Autodesk Inventor part; units mm, degrees
ref_plane "YZ Plane" through (0, 0, 0) normal (1, 0, 0) x (0, 1, 0)
ref_plane "XZ Plane" through (0, 0, 0) normal (0, 1, 0) x (-1, 0, 0)
ref_plane "XY Plane" through (0, 0, 0) normal (0, 0, 1) x (1, 0, 0)
sketch "Sketch1" plane through (0, 0, 0) normal (0, 0, 1) x (1, 0, 0)
  circle A0 centre (0, 0) radius 45.212
  dimension "d0" = 90.424
extrude "Extrusion1" add sketch "Sketch1" along normal blind 4.7625
sketch "Sketch6" plane through (0, 0, 4.7625) normal (0, 0, 1) x (1, 0, 0)
  circle A0 centre (12.446, -29.7561) radius 3.048
  point P0 (0, 0)
  dimension "d27" = 6.096
  dimension "d28" = 29.7561
  dimension "d29" = 12.446
extrude "Extrusion6" cut sketch "Sketch6" against normal blind 25.4
sketch "Sketch7" plane through (0, 0, 4.7625) normal (0, 0, 1) x (1, 0, 0)
  line L0 (0, 0) -> (21.4313, 37.12)
  line L1 (0, 0) -> (42.8625, 0) construction
  circle A0 centre (21.4313, 37.12) radius 1.7145
  circle A1 centre (-21.4312, 37.12) radius 1.7145
  circle A2 centre (-42.8625, 0) radius 1.7145
  circle A3 centre (-21.4313, -37.12) radius 1.7145
  circle A4 centre (21.4312, -37.12) radius 1.7145
  circle A5 centre (42.8625, 0) radius 1.7145
  dimension "d32" = 42.8625
  dimension "d33" = 60
  dimension "d34" = 3.429
  dimension "d37" = 360
extrude "Extrusion7" cut sketch "Sketch7" against normal blind 25.4
sketch "Sketch8" plane through (0, 0, 4.7625) normal (0, 0, 1) x (1, 0, 0)
  line L0 (0, 0) -> (0, 41.91)
  circle A0 centre (0, 41.91) radius 1.8415
  circle A1 centre (-36.2951, 20.955) radius 1.8415
  circle A2 centre (-36.2951, -20.955) radius 1.8415
  circle A3 centre (0, -41.91) radius 1.8415
  circle A4 centre (36.2951, -20.955) radius 1.8415
  circle A5 centre (36.2951, 20.955) radius 1.8415
  dimension "d41" = 41.91
  dimension "d42" = 3.683
  dimension "d45" = 360
extrude "Extrusion8" cut sketch "Sketch8" against normal blind 25.4
sketch "Sketch10" plane through (0, 0, 4.7625) normal (0, 0, 1) x (1, 0, 0)
  line L0 (0, 0) -> (39.3779, 10.5513)
  line L1 (0, 0) -> (40.767, 0) construction
  circle A0 centre (39.3779, 10.5513) radius 3.81
  line L2 (0, 0) -> (0, 16.2318)
  circle A1 centre (39.3779, -10.5513) radius 3.81
  circle A2 centre (-39.3779, 10.5513) radius 3.81
  circle A3 centre (-39.3779, -10.5513) radius 3.81
  line L3 (0, 0) -> (28.8266, 28.8266)
  line L4 (0, 0) -> (40.767, 0) construction
  circle A4 centre (28.8266, 28.8266) radius 3.81
  circle A5 centre (-28.8266, 28.8266) radius 3.81
  dimension "d49" = 40.767
  dimension "d50" = 15
  dimension "d51" = 7.62
  dimension "d68" = 40.767
  dimension "d69" = 45
  dimension "d70" = 7.62
extrude "Extrusion9" cut sketch "Sketch10" against normal blind 25.4 contours A0 | A1 | A2 | A3
sketch "Sketch11" plane through (0, 0, 4.7625) normal (0, 0, 1) x (1, 0, 0)
  circle A0 centre (-39.3779, 10.5513) radius 3.81
  circle A1 centre (39.3779, 10.5513) radius 3.81
  circle A2 centre (39.3779, -10.5513) radius 3.81
  circle A3 centre (-39.3779, -10.5513) radius 3.81
  circle A4 centre (36.2951, -20.955) radius 1.8415
  circle A5 centre (-36.2951, -20.955) radius 1.8415
  circle A6 centre (0, 41.91) radius 1.8415
  circle A7 centre (-36.2951, 20.955) radius 1.8415
  circle A8 centre (0, -41.91) radius 1.8415
  circle A9 centre (36.2951, 20.955) radius 1.8415
  circle A10 centre (21.4312, -37.12) radius 1.7145
  circle A11 centre (-42.8625, 0) radius 1.7145
  circle A12 centre (21.4313, 37.12) radius 1.7145
  circle A13 centre (-21.4312, 37.12) radius 1.7145
  circle A14 centre (-21.4313, -37.12) radius 1.7145
  circle A15 centre (42.8625, 0) radius 1.7145
  circle A16 centre (12.446, -29.7561) radius 3.048
  circle A17 centre (0, 0) radius 45.212
  circle A18 centre (0, 0) radius 25.4
  dimension "d54" = 50.8
extrude "Extrusion10" cut sketch "Sketch11" against normal blind 25.4 contours A18
sketch "Sketch12" plane through (0, 0, 4.7625) normal (0, 0, 1) x (1, 0, 0)
  circle A0 centre (0, 0) radius 25.4
  circle A1 centre (-39.3779, 10.5513) radius 3.81
  circle A2 centre (39.3779, 10.5513) radius 3.81
  circle A3 centre (39.3779, -10.5513) radius 3.81
  circle A4 centre (-39.3779, -10.5513) radius 3.81
  circle A5 centre (36.2951, -20.955) radius 1.8415
  circle A6 centre (-36.2951, -20.955) radius 1.8415
  circle A7 centre (0, 41.91) radius 1.8415
  circle A8 centre (-36.2951, 20.955) radius 1.8415
  circle A9 centre (0, -41.91) radius 1.8415
  circle A10 centre (36.2951, 20.955) radius 1.8415
  circle A11 centre (21.4312, -37.12) radius 1.7145
  circle A12 centre (-42.8625, 0) radius 1.7145
  circle A13 centre (21.4313, 37.12) radius 1.7145
  circle A14 centre (-21.4312, 37.12) radius 1.7145
  circle A15 centre (-21.4313, -37.12) radius 1.7145
  circle A16 centre (42.8625, 0) radius 1.7145
  circle A17 centre (12.446, -29.7561) radius 3.048
  circle A18 centre (0, 0) radius 45.212
  circle A19 centre (0, 0) radius 33.3375
  line L0 (0, 0) -> (0, -33.3375)
  line L1 (0, 0) -> (12.446, -29.7561)
  line L2 (0, 0) -> (23.7355, -23.4097)
  line L3 (0, -25.4) -> (0, -33.3375)
  line L4 (18.0842, -17.836) -> (23.7355, -23.4097)
  arc A20 (0, -25.4) -> (18.0842, -17.836) centre (0, 0) ccw
  arc A21 (0, -33.3375) -> (23.7355, -23.4097) centre (0, 0) ccw
  dimension "d57" = 66.675
extrude "Extrusion11" cut sketch "Sketch12" against normal blind 25.4 contours A0 L0 A19 L2
fillet "Fillet2" radius 3.175 2 edges at (23.7355, -23.4097, 2.3813) (0, -33.3375, 2.3813)
sketch "Sketch14" plane through (0, 0, 4.7625) normal (0, 0, 1) x (1, 0, 0)
  circle A0 centre (0, 0) radius 45.212
  circle A1 centre (12.446, -29.7561) radius 3.048
  circle A2 centre (42.8625, 0) radius 1.7145
  circle A3 centre (-21.4313, -37.12) radius 1.7145
  circle A4 centre (-21.4312, 37.12) radius 1.7145
  circle A5 centre (21.4313, 37.12) radius 1.7145
  circle A6 centre (-42.8625, 0) radius 1.7145
  circle A7 centre (21.4312, -37.12) radius 1.7145
  circle A8 centre (36.2951, 20.955) radius 1.8415
  circle A9 centre (0, -41.91) radius 1.8415
  circle A10 centre (-36.2951, 20.955) radius 1.8415
  circle A11 centre (0, 41.91) radius 1.8415
  circle A12 centre (-36.2951, -20.955) radius 1.8415
  circle A13 centre (36.2951, -20.955) radius 1.8415
  circle A14 centre (-39.3779, -10.5513) radius 3.81
  circle A15 centre (39.3779, -10.5513) radius 3.81
  circle A16 centre (39.3779, 10.5513) radius 3.81
  circle A17 centre (-39.3779, 10.5513) radius 3.81
  line L0 (0, -25.4) -> (0, -29.9949)
  arc A18 (-3.5092, -33.1523) -> (0, -29.9949) centre (-3.175, -29.9949) ccw
  arc A19 (26.0678, -20.7812) -> (-3.5092, -33.1523) centre (0, 0) ccw
  arc A20 (21.3557, -21.0626) -> (26.0678, -20.7812) centre (23.5852, -18.802) ccw
  line L1 (21.3557, -21.0626) -> (18.0842, -17.836)
  line L2 (24.2654, 22.86) -> (-24.2654, 22.86)
  arc A21 (0, -25.4) -> (18.0842, -17.836) centre (0, 0) ccw
  dimension "d64" = 22.86
extrude "Extrusion13" add sketch "Sketch14" against normal up to surface (4.7625 mm away) contours A19 L2
fillet "Fillet3" radius 3.175 2 edges at (24.2654, 22.86, 2.3813) (-24.2654, 22.86, 2.3813)
extrude "Extrusion14" cut sketch "Sketch10" against normal blind 25.4 contours A4 | A5
sketch "Sketch16" plane through (0, 0, 4.7625) normal (0, 0, 1) x (1, 0, 0)
  circle A0 centre (-7.9375, 29.1338) radius 3.048
  point P0 (0, 0)
  dimension "d73" = 6.096
  dimension "d74" = 7.9375
  dimension "d75" = 29.1338
extrude "Extrusion15" cut sketch "Sketch16" against normal through all
fillet "Fillet4" radius 12.7 2 edges at (18.0842, -17.836, 2.3813) (0, -25.4, 2.3813)
properties part number "AluminumSealingDiscMidshipsRear" material "Aluminum 6061"
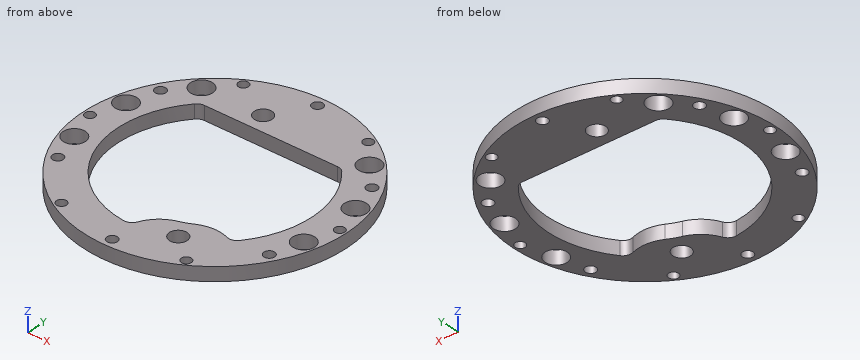
Geometry check sheet. Reference: the model listing, model coordinates, mm. Give positions to 0.01 mm unless a question says otherwise; leave off trailing zeros. Write each loop counter-clockwise with the first axis right and the second up, starting at its lowest first coordinate (ties: lowest second). Pieces come first, ordered by that corner, then holes.
1) Section check A-A, the plane y = 0. Record the boundary of the cut face in (x, z), and give its area (3 significant figures).
2) Section check D-D, the plane z = 1.15. State how many separate pieces and enclosed holes the cut face has, and give its area (3 significant figures).
3) Gauge pin test, flat ends, axial feed: pin 1 (3 mm diameter, centred on x = -9, y = -31.5, fed in from +Z); pin 2 (2 mm diameter, centred on y = -21.5, z = 2, fed in from +X). Record the tip position at first contact, or that the pin passes through.
4) Section check C-C, the plane x = -16. Record the boundary of the cut face in (y, z), and give its area (3 significant figures).
5) Material ranges on L1, parallel to Y at x = -39, z = 4.25; L2, parallel to X at y = 9.5, z = 0.8; L3, parallel to Y at x = 41, z = 1.4, recorded low to high.
6) Section check B-B, the plane y = 41.91. Record the boundary of the cut face in (x, z), and give its area (3 significant figures).
Computed:
1. outline: (-45.21, 0) - (-44.58, 0) - (-44.58, 4.76) - (-45.21, 4.76) - close; (-41.15, 0) - (-33.34, 0) - (-33.34, 4.76) - (-41.15, 4.76) - close; (33.34, 0) - (41.15, 0) - (41.15, 4.76) - (33.34, 4.76) - close; (44.58, 0) - (45.21, 0) - (45.21, 4.76) - (44.58, 4.76) - close
1. area: 80.4 mm2
2. separate pieces: 1
2. enclosed holes: 21
2. area: 3,000 mm2
3. pin 1: stops at z = 4.76
3. pin 2: stops at x = 40.3
4. outline: (-42.29, 0) - (-29.25, 0) - (-29.25, 4.76) - (-42.29, 4.76) - close; (22.86, 0) - (42.29, 0) - (42.29, 4.76) - (22.86, 4.76) - close
4. area: 155 mm2
5. L1: y = -22.87 to -14.34, -6.76 to 6.76, 14.34 to 22.87
5. L2: x = -44.2 to -43.04, -35.72 to -31.96, 31.96 to 35.72, 43.04 to 44.2
5. L3: y = -19.06 to -14, -7.1 to 7.1, 14 to 19.06
6. outline: (-16.96, 0) - (-1.84, 0) - (-1.84, 4.76) - (-16.96, 4.76) - close; (1.84, 0) - (16.96, 0) - (16.96, 4.76) - (1.84, 4.76) - close
6. area: 144 mm2
